Source: CAD feature listing. Evaluate the final solid. Frame: model axes, mm. A direction names the side the tool comes from. Give positions to 0.01 mm unless a question says otherwise; leave off trailing zeros. Order: outer loops, then holes, each group sorted by start corner. A loop starts at its lowest first (then second) coordinate and runs counter-clockwise, first axis right, second up. Notation, with made-up numbers: M 81,32 L 114,32 A11 ccw 114,39 Z; hole C -33.5,84.25 d6. An arc over 180 degrees is marked long. Answer in a Markdown table with one row per item. Add a question column.
(1) Material intervals for line 1 along Z through (x, y) = (1, 15.87); line 2 along Z through (x, y) = (19.05, 1.3) (3 decimals); line 3 along X through (y, z) = (19, -57.5) (3 decimals), sorted ascending.
(2) Pin query (flat end, axial travel): P1, Ø3.5, axis at x = 19.05, z = -53.975, coming from the +Y side; P2, Ø7, axis at y = 19.05, z = 53.975, coming from the +X side (3 decimals); P3, Ø7, axis at x = 15.87, z = -38.1, coming from the +Y side (3 decimals). Return the tip coordinate at first contact, or that it passes through.
(3) Section query B-B, the plane y = 19.75. Return loops of the section in (x, z) (3 decimals).
(4) Section query C-C, the plane z = 45. Return loops of the section in (x, y) (3 decimals), plus the area to 3 significant figures.
(5) Section query D-D, the plane y = 10.75. Return loops of the section in (x, z) (3 decimals).
(6) Mould query, pull axis Y, two halves, no side actions, for faces 1 (the face through (1.565, 18.016, 0.676)), 2 (the face through (2, 25.4, 1)), 3 (the face through (25.4, 2, 1)), 4 (the face through (1.565, 10.096, -62.521)). Classes: pulls with the +Y half, pulls with the -Y half, needs draft (parallel to the pull), parting line crosses it, or undercut.
(7) Section query A-A, the plane z = -38.1. Return loops of the section in (x, y) (3 decimals).
(8) Set-up query: faces 5 (the face through (18.1, 3.175, 0.9)), 6 (the face through (17.26, 1.57, -55.34)). Return all of +Z, -Z, +X, -X, +Y, -Y with unobstructed straight access to the full face (end or side cutting, diameter ignored); none if empty.
from build123d import *

# Parameters (mm, degrees)
BOSS_EXTRUDE1_DEPTH = 63.5
FILLET1_R           = 3.175
SKETCH2_R           = 2.25
CUT_EXTRUDE1_DEPTH  = 26.4


with BuildPart() as part:
    # Sketch1 → Boss-Extrude1 (new body, symmetric)
    with BuildSketch(Plane.XY):
        Polygon((0, 25.4), (0, 0), (25.4, 0), (25.4, 3.175), (3.175, 3.175), (3.175, 25.4), align=None)
    extrude(amount=BOSS_EXTRUDE1_DEPTH, both=True)

    # Fillet1
    fillet1_edges = [part.edges().sort_by_distance(p)[0] for p in [
        (3.175, 3.175, 0),
    ]]
    fillet(fillet1_edges, radius=FILLET1_R)

    # Sketch2 → Cut-Extrude1 (cut, through all)
    with BuildSketch(Plane.XZ):
        with Locations((19.05, -53.975)):
            Circle(SKETCH2_R)
        with Locations((10.583333333, -60.325)):
            Circle(SKETCH2_R)
        with Locations((10.583333333, 60.325)):
            Circle(SKETCH2_R)
        with Locations((19.05, 53.975)):
            Circle(SKETCH2_R)
        with Locations((15.87, 38.1)):
            Circle(SKETCH2_R)
        with Locations((15.87, 0)):
            Circle(SKETCH2_R)
        with Locations((15.87, -38.1)):
            Circle(SKETCH2_R)
    cut_extrude1 = extrude(amount=-CUT_EXTRUDE1_DEPTH, mode=Mode.SUBTRACT)

    # Mirror1: Cut-Extrude1 across plane
    add(cut_extrude1.mirror(Plane(origin=(0, 0, 0), x_dir=(0, 0, 1), z_dir=(0.707106781, -0.707106781, 0))), mode=Mode.SUBTRACT)


solid = part.part
Values follow:
| question | item | result |
|---|---|---|
| 1 | line 1 | z = -63.5 to -40.35, -35.85 to -2.25, 2.25 to 35.85, 40.35 to 63.5 |
| 1 | line 2 | z = -63.5 to -56.225, -51.725 to 51.725, 56.225 to 63.5 |
| 1 | line 3 | x = 0 to 3.175 |
| 2 | P1 | passes through |
| 2 | P2 | stops at x = 3.175 |
| 2 | P3 | stops at y = 3.175 |
| 3 | outline | M 0,-63.5 L 3.175,-63.5 L 3.175,-56.113 L 0,-56.113 Z; M 0,-51.837 L 3.175,-51.837 L 3.175,51.837 L 0,51.837 Z; M 0,56.113 L 3.175,56.113 L 3.175,63.5 L 0,63.5 Z |
| 4 | outline | M 0,0 L 25.4,0 L 25.4,3.175 L 6.35,3.175 A3.175 cw 3.175,6.35 L 3.175,25.4 L 0,25.4 Z |
| 4 | area | 153 mm² |
| 5 | outline | M 0,-63.5 L 3.175,-63.5 L 3.175,-62.569 L 0,-62.569 Z; M 0,-58.081 L 3.175,-58.081 L 3.175,58.081 L 0,58.081 Z; M 0,62.569 L 3.175,62.569 L 3.175,63.5 L 0,63.5 Z |
| 6 | face 1 | undercut |
| 6 | face 2 | pulls with the +Y half |
| 6 | face 3 | needs draft |
| 6 | face 4 | undercut |
| 7 | outline | M 0,0 L 13.62,0 L 13.62,3.175 L 6.35,3.175 A3.175 cw 3.175,6.35 L 3.175,13.62 L 0,13.62 Z; M 0,18.12 L 3.175,18.12 L 3.175,25.4 L 0,25.4 Z; M 18.12,0 L 25.4,0 L 25.4,3.175 L 18.12,3.175 Z |
| 8 | face 5 | +Z, -Z, +X, +Y |
| 8 | face 6 | +Y, -Y |
